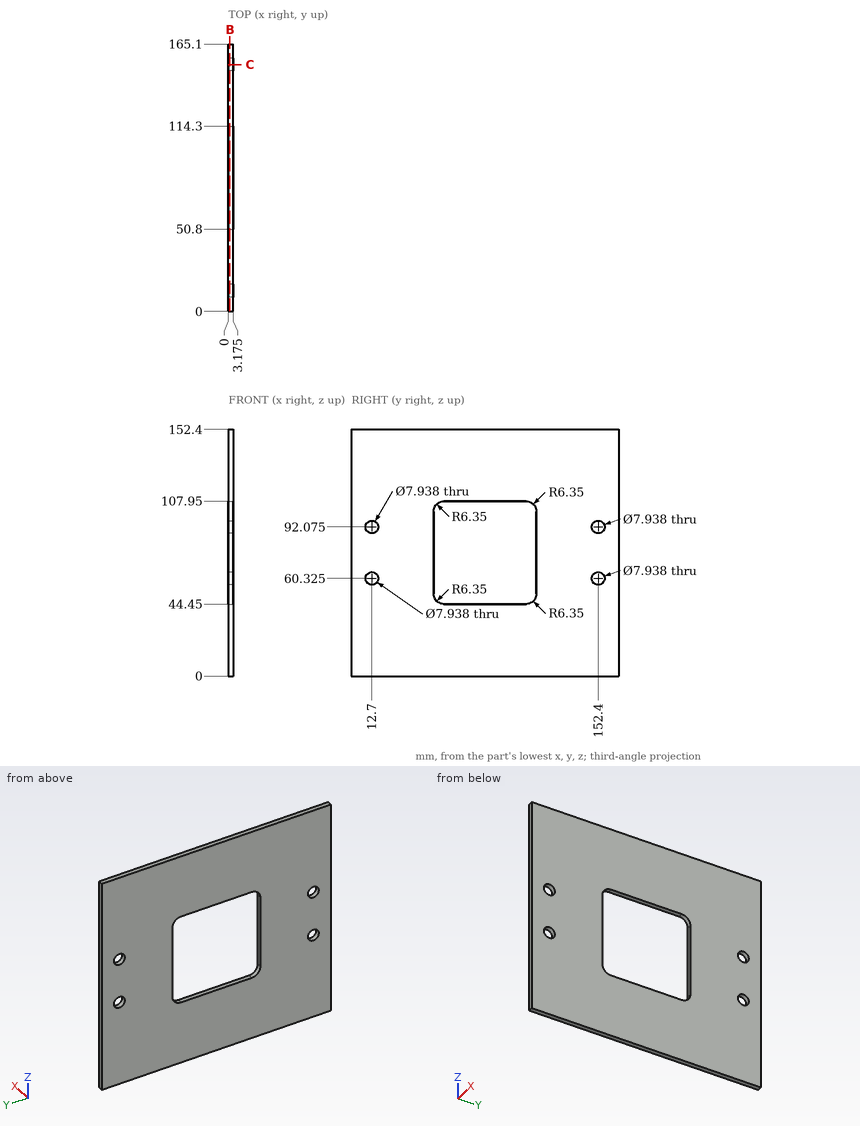
The figure shows three views and two pictorial views of one solid part (mm, origin at its lowest corner). Answer the questions. Give positions to 0.01 mm unless a question says otherwise; leave off trailing zeros. Loops run counter-clockwise (first coordinate to the right, second up) from the corner with the lowest first, then second, coordinate; pieces in that order, holes last. Notation, with made-up numbers: (89.25, 49) -> (122.25, 49) arc R29 ccw to (122.25, 78) -> close; hole circle Ø3 at (32.25, -34.75). An arc over 180 degrees is marked (long way). Put each result on its own line as item: value. Start each with the question number.
Item 1: The part is cut by section B-B (x = 0.9). State how many separate pieces and enclosed holes the cut face has, then the cut area to 3 significant figures.
Item 2: The part is cut by section C-C (y = 152.4). Give the vertices of the cut face in (x, z) (1 decimal).
Item 3: Each of these flat-tipped pins is pushed along its axis until it touches: P1, Ø6, axis at y = 131, z = 56, coming from the -X side; P2, Ø6.5, axis at y = 12.7, z = 60.325, coming from the +X side. Where does it stop, or does it pass through?
Item 4: Find the intervals of material crossed by L1, parallel to Z at x = 0.7, y = 152.4; L2, parallel to Z at x = 1.6, y = 96; L3, parallel to Y at x = 0.55, z = 89.5, in increasing order. Write a range as [from, to].
Answers below:
1. separate pieces: 1
1. enclosed holes: 5
1. area: 21,000 mm2
2. outline: (0, 0) -> (3.2, 0) -> (3.2, 56.4) -> (0, 56.4) -> close; (0, 64.3) -> (3.2, 64.3) -> (3.2, 88.1) -> (0, 88.1) -> close; (0, 96) -> (3.2, 96) -> (3.2, 152.4) -> (0, 152.4) -> close
3. P1: x = 0
3. P2: through
4. L1: [0, 56.36], [64.29, 88.11], [96.04, 152.4]
4. L2: [0, 44.45], [107.95, 152.4]
4. L3: [0, 9.68], [15.72, 50.8], [114.3, 149.38], [155.42, 165.1]
